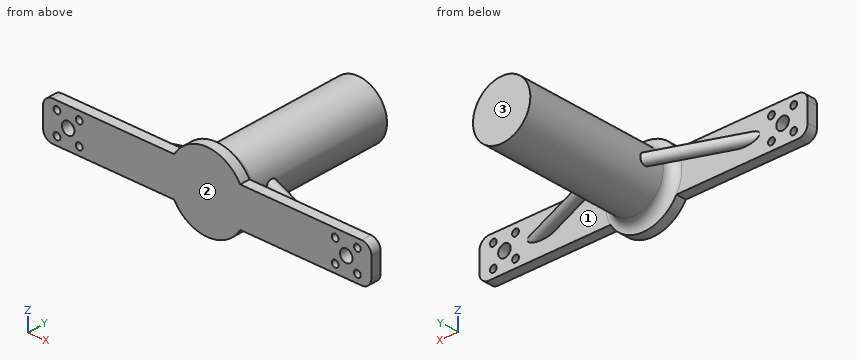
```python
from build123d import *

# Parameters (mm, degrees)
BOSS_EXTRUDE1_DEPTH = 5.25
SKETCH3_R           = 14.850000000000001
BOSS_EXTRUDE2_DEPTH = 80
SKETCH2_R           = 1.749999999999997
SKETCH2_R_2         = 3.250000000000007
CUT_EXTRUDE1_DEPTH  = 119.39358090707452
FILLET8_R           = 5
FILLET9_R           = 5


with BuildPart() as part:
    # Sketch1 → Boss-Extrude1 (new body)
    with BuildSketch(Plane(origin=(0, 0, 0), x_dir=(1, 0, 0), z_dir=(0, 1, 0))):
        with BuildLine():
            Line((-85, -10.000000000000002), (-17.089177862027185, -10))
            ThreePointArc((-17.089177862027185, -10), (1.11e-15, -19.8), (17.089177862027185, -10))
            Line((17.089177862027185, -10), (85, -10.000000000000002))
            Line((85, -10.000000000000002), (85, 10))
            Line((85, 10), (17.089177862027185, 10))
            ThreePointArc((17.089177862027185, 10), (1.11e-15, 19.8), (-17.089177862027185, 10))
            Line((-17.089177862027185, 10), (-85, 10))
            Line((-85, 10), (-85, -10.000000000000002))
        make_face()
    extrude(amount=BOSS_EXTRUDE1_DEPTH)

    # Sketch3 → Boss-Extrude2 (add)
    with BuildSketch(Plane(origin=(0, 5.25, 0), x_dir=(1, 0, 0), z_dir=(0, 1, 0))):
        with Locations(Location((0, 0, 0), (0, 0, 270))):
            Circle(SKETCH3_R)
    extrude(amount=BOSS_EXTRUDE2_DEPTH)

    # Sketch2 → Cut-Extrude1 (cut, through all)
    with BuildSketch(Plane(origin=(0, 5.25, 0), x_dir=(1, 0, 0), z_dir=(0, 1, 0))):
        with Locations(Location((-77.75, 5.7499999999999964, 0), (0, 0, 270))):
            Circle(SKETCH2_R)
        with Locations(Location((-66.25, 5.7499999999999964, 0), (0, 0, 270))):
            Circle(SKETCH2_R)
        with Locations(Location((-66.25, -5.75, 0), (0, 0, 270))):
            Circle(SKETCH2_R)
        with Locations(Location((-77.75, -5.75, 0), (0, 0, 270))):
            Circle(SKETCH2_R)
        with Locations(Location((77.75, -5.75, 0), (0, 0, 270))):
            Circle(SKETCH2_R)
        with Locations(Location((66.25, -5.75, 0), (0, 0, 270))):
            Circle(SKETCH2_R)
        with Locations(Location((77.75, 5.7499999999999964, 0), (0, 0, 270))):
            Circle(SKETCH2_R)
        with Locations(Location((66.25, 5.7499999999999964, 0), (0, 0, 270))):
            Circle(SKETCH2_R)
        with Locations(Location((-72, -2.87e-15, 0), (0, 0, 270))):
            Circle(SKETCH2_R_2)
        with Locations(Location((72, -2.87e-15, 0), (0, 0, 270))):
            Circle(SKETCH2_R_2)
    extrude(amount=-CUT_EXTRUDE1_DEPTH, mode=Mode.SUBTRACT)

    # Sketch5 one side → Revolve1 (revolve)
    with BuildSketch(Plane.XY, mode=Mode.PRIVATE) as revolve1_sk:
        Polygon((-14.850000000000001, 20.23639427704437), (-14.850000000000001, 23.25), (-60.077367189450115, 5.2500000000000036), (-59.041984669000975, 2.648465253672675), align=None)
    revolve1 = revolve(revolve1_sk.sketch.rotate(Axis((-59.041984669000975, 2.648465253672677, 0), (0.9291195522597585, 0.3697794715889807, 0)), 180), axis=Axis((-59.041984669000975, 2.648465253672677, 0), (0.9291195522597585, 0.3697794715889807, 0)))

    # Fillet8
    fillet8_edges = [part.edges().sort_by_distance(p)[0] for p in [
        (85, 2.625, -10),
        (85, 2.625, 10.000000000000002),
        (-85, 2.625, 10.000000000000002),
        (-85, 2.625, -10),
    ]]
    fillet(fillet8_edges, radius=FILLET8_R)

    # Mirror1: Revolve1 across plane
    add(revolve1.mirror(Plane.ZY))

    # Fillet9
    # the kernel refuses this fillet: 5 mm, written as the material it adds along each edge
    with BuildSketch(Plane(origin=(0, 5.25, 0), x_dir=(-1.8e-16, 0, 1), z_dir=(-1, 0, -1.8e-16))) as fillet9_piece_1:
        with BuildLine():
            CenterArc((19.85, 4.99974999375026), FILLET9_R, 180, 89.42703265514302)
            Line((14.850000000000001, 4.99974999375026), (14.750000000000002, 4.99974999375026))
            Line((14.750000000000002, 4.99974999375026), (14.750000000000002, 0))
            Line((14.750000000000002, 0), (14.850000000000001, -0.09999999999999964))
            ThreePointArc((14.850000000000001, -0.09999999999999964), (17.32500000000001, -0.09999999999999964), (19.799000000000017, -0.09999499987442118))
            Line((19.799000000000017, -0.09999499987442118), (19.80000000000002, 5.7288e-13))
        make_face()
    revolve(axis=Axis((0, 5.25, 0), (0, 1, 0)))


solid = part.part
```
Input: part model. Units: mm. Frame: model coordinates. Face numbers are marked on the shaded views. Round coordinates to 2 decimals unless told otherwise and drop trailing zeros. Write each loop counter-clockwise with the first axis right and the second up, starting at its lowest first coordinate (ties: lowest second). Pieces come first, ordered by that corner, then holes. Notation, with made-up numbers: (6.5, 3) - (49.5, 3) arc R13 cw to (49.5, 18) - close; hole circle Ø3 at (60.5, -6). An arc over 180 degrees is marked (long way). Write item = value, one per line.
(1) Section query D-D on y = 77. Output: boundary loops of the cut face in (x, z), then the cut area to 3 significant figures.
Geometry check:
outline = circle Ø29.7 at (0, 0)
area = 693 mm^2
(2) Material intervals for probe 1 along X at (y, z) = (2.1, 0); probe 2 along Z at (x, y) = (-66.25, 2.6); probe 3 along X at (y, z) = (1.7, -5.75), sorted ascending.
Geometry check:
probe_1 = -85 to -75.25, -68.75 to 68.75, 75.25 to 85
probe_2 = -10 to -7.5, -4 to 4, 7.5 to 10
probe_3 = -84.94 to -79.5, -76 to -68, -64.5 to 64.5, 68 to 76, 79.5 to 84.94
(3) Section query C-C on x = 0. Output: boundary loops of the cut face in (y, z), then the cut area to 3 significant figures.
Geometry check:
outline = (0, -19.8) - (5.25, -19.8) arc R5 cw to (10.25, -14.85) - (85.25, -14.85) - (85.25, 14.85) - (10.25, 14.85) arc R5 cw to (5.25, 19.8) - (0, 19.8) - close
area = 2,590 mm^2
(4) Pull-direction query (Y, two-part tool) for the marked faces 1, 2 and 3; classes: +Y half, -Y half, draft (parallel to the pull), parting line (faces both ways), or undercut.
Geometry check:
face_1 = undercut
face_2 = -Y half
face_3 = +Y half
(5) Section query A-A on x = -66.25. Output: boundary loops of the cut face in (y, z).
Geometry check:
outline = (0, -10) - (5.25, -10) - (5.25, -7.5) - (0, -7.5) - close; (0, -4) - (5.25, -4) - (5.25, 4) - (0, 4) - close; (0, 7.5) - (5.25, 7.5) - (5.25, 10) - (0, 10) - close
(6) Section query B-B on z = 0. Output: boundary loops of the cut face in (x, y), then the cut area to 3 significant figures.
Geometry check:
outline = (-85, 0) - (-75.25, 0) - (-75.25, 5.25) - (-85, 5.25) - close; (-68.75, 0) - (68.75, 0) - (68.75, 5.25) - (60.08, 5.25) - (14.85, 23.25) - (14.85, 85.25) - (-14.85, 85.25) - (-14.85, 23.25) - (-60.08, 5.25) - (-68.75, 5.25) - close; (75.25, 0) - (85, 0) - (85, 5.25) - (75.25, 5.25) - close; hole (-44.93, 5.25) - (-19.8, 5.25) arc R5 ccw to (-14.85, 10.25) - (-14.85, 17.22) - close; hole (14.85, 10.25) arc R5 ccw to (19.8, 5.25) - (44.93, 5.25) - (14.85, 17.22) - close
area = 3,660 mm^2
(7) Contact query for flat-ended pins moving along their axis: pin 1 Ø4.5 at (x, z) = (77.75, -5.75) entering from +Y; pin 2 Ø6 at (y, z) = (55, 15.5) entering from +X; pin 3 Ø4.5 at (x, z) = (-66.25, 5.75) entering from +Y. Output: stop coordinate, or through.
Geometry check:
pin_1 = 5.25
pin_2 = 8.02
pin_3 = 5.25
